Check sheet for the modelled part. Datum: model origin and axes. Units: mm. A direction names the side the tool comes from. Give positions to 0.01 mm unless a question says otherwise; leave off trailing zeros. Loops run counter-clockwise (first coordinate to the right, second up) from the corner with the lowest first, then second, coordinate; pieces in that order, holes last. Notation, with made-up numbers: (17.25, -23.75) - (55.25, -23.75) arc R15 cw to (55.25, -15.75) - close; hole circle Ø1 at (61, 30). An arc over 180 degrees is marked (long way). Answer in a Markdown table with one row per item. Add a question column.
(1) Sectioned sample at D-D on z = 11.25. Enter the section's corners in (x, y).
(2) Sectioned sample at C-C on y = -0.5. Enter the section's corners in (x, z), then the cut area to 3 significant figures.
(3) Sectioned sample at B-B on x = 0. Enter the section's corners in (y, z), then the cut area to 3 significant figures.
(4) Set-up check for faces 1 (the face through (0.6, 0, -1)), 2 (the face through (-2.4, 0, 2)): record each of +Z, -Z, +X, -X, +Y, -Y from which the full face is reachable in a straight line by a thin tool's end or side.
(5) Thickness scan on L1, parallel to Y at x = 0, z = 8; L2, parallel to Y at x = -2.75, z = 1.5; L3, parallel to Y at x = 3.5, z = 13. Record the ranges inside material, lowest first.
(6) Sectioned sample at A-A on z = 1.5. Enter the section's corners in (x, y).
(7) Go/stop test with flat-tipped pins: P1, Ø0.6, axis at x = 0.5, z = -0.5, coming from the +Y side; P2, Ø0.6, axis at x = 2.5, z = 1.5, coming from the -Y side; P3, Ø0.9, axis at x = 2.5, z = 1.5, coming from the +Y side. Record where each tip stops, or that it passes through.
(8) Draft check along Y on faces 3 (the face through (-1.08, -4.88, 6.87)), 4 (the face through (1, 0, -1.5)), 5 (the face through (2.8, 0, 1)). Enter one of: released by +Y, released by -Y, zero draft, split by the parting line, or undercut.
from build123d import *

# Parameters (mm, degrees)
F0_R     = 5
F0_R_2   = 4
F1_DEPTH = 15
F2_R     = 5
F3_DEPTH = 1.5
F4_W     = 1.2
F4_H     = 6.4
F5_DEPTH = 2
F6_W     = 0.8
F6_H     = 4
F7_DEPTH = 2


# Not quite as in the source:
# - a pattern or mirror of a feature is missing from the dataset's text; its kind, count and spacing are read off the source's solid


with BuildPart() as f1:
    # F0 (on Top) → F1 (new body)
    with BuildSketch(Plane.XY):
        Circle(F0_R)
        Circle(F0_R_2, mode=Mode.SUBTRACT)
    extrude(amount=F1_DEPTH)

    # F2 (on Top) → F3 (join)
    with BuildSketch(Plane.XY):
        Circle(F2_R)
    extrude(amount=-F3_DEPTH)

    # F4 (on Top) → F5 (cut)
    with BuildSketch(Plane.XY):
        Rectangle(F4_W, F4_H)
    extrude(amount=-F5_DEPTH, mode=Mode.SUBTRACT)

    # F6 (on Top) → F7 (join)
    with BuildSketch(Plane.XY):
        with Locations((2.4, 0)):
            Rectangle(F6_W, F6_H)
    f7 = extrude(amount=F7_DEPTH)

    # F7_copies: F7 across plane
    add(f7.mirror(Plane(origin=(0, 0, 0), x_dir=(0, 0, -1), z_dir=(-1, 0, 0))))


solid = f1.part
Reply:
| question | item | result |
|---|---|---|
| 1 | outline | circle Ø10 at (0, 0); hole circle Ø8 at (0, 0) |
| 2 | outline | (-4.97, -1.5) - (-0.6, -1.5) - (-0.6, 0) - (-2, 0) - (-2, 2) - (-2.8, 2) - (-2.8, 0) - (-3.97, 0) - (-3.97, 15) - (-4.97, 15) - close; (0.6, -1.5) - (4.97, -1.5) - (4.97, 15) - (3.97, 15) - (3.97, 0) - (2.8, 0) - (2.8, 2) - (2, 2) - (2, 0) - (0.6, 0) - close |
| 2 | area | 46.5 mm^2 |
| 3 | outline | (-5, -1.5) - (-3.2, -1.5) - (-3.2, 0) - (-4, 0) - (-4, 15) - (-5, 15) - close; (3.2, -1.5) - (5, -1.5) - (5, 15) - (4, 15) - (4, 0) - (3.2, 0) - close |
| 3 | area | 35.4 mm^2 |
| 4 | face 1 | +Z, -Z |
| 4 | face 2 | +Z |
| 5 | L1 | -5 to -4, 4 to 5 |
| 5 | L2 | -4.18 to -2.9, -2 to 2, 2.9 to 4.18 |
| 5 | L3 | -3.57 to -1.94, 1.94 to 3.57 |
| 6 | outline | circle Ø10 at (0, 0); (-2.8, -2) - (-2, -2) - (-2, 2) - (-2.8, 2) - close; (2, -2) - (2.8, -2) - (2.8, 2) - (2, 2) - close; hole circle Ø8 at (0, 0) |
| 7 | P1 | y = 5 |
| 7 | P2 | y = -4.49 |
| 7 | P3 | y = 4.56 |
| 8 | face 3 | split by the parting line |
| 8 | face 4 | zero draft |
| 8 | face 5 | undercut |
